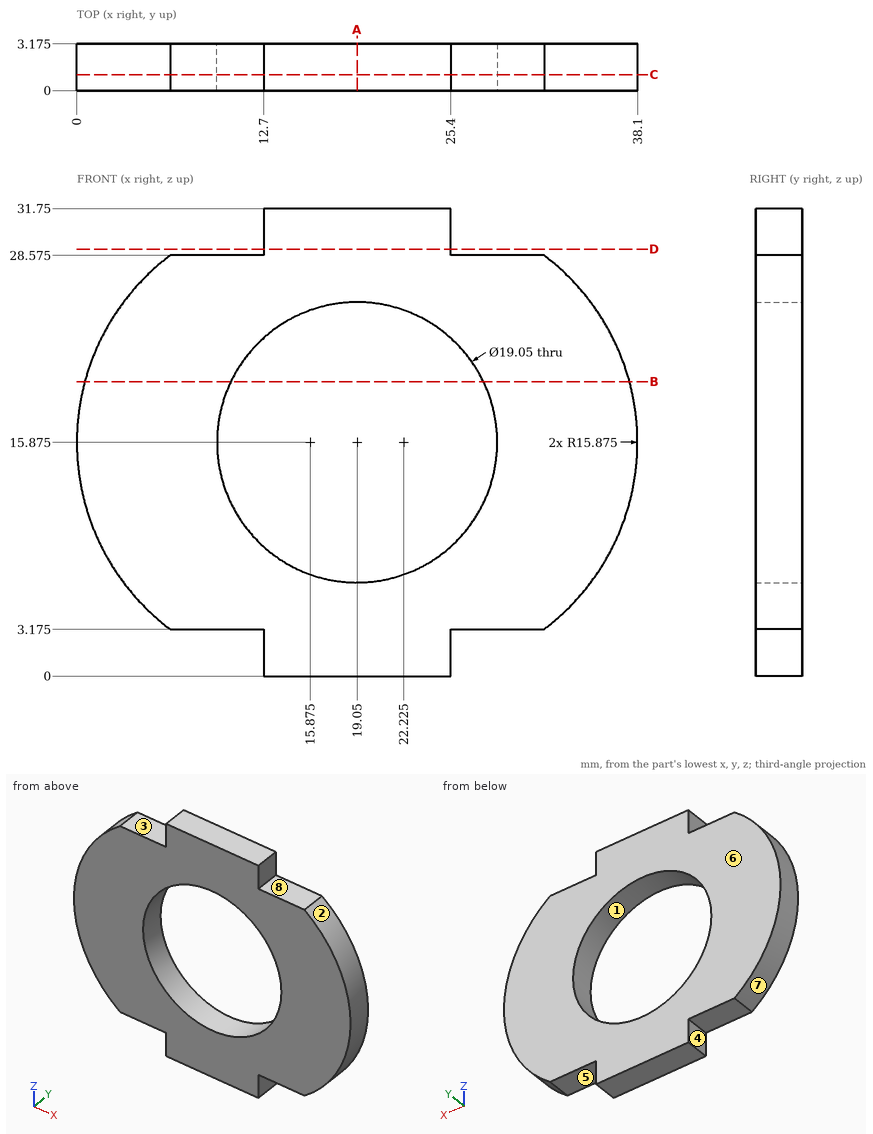
The drawing under review shows one solid part. Ordinate dimensions are in mm from its lowest x, y, z. A direction names the side the tool comes from. Coordinates: 2 decimals unless noted, no trailing zeros. Write each loop counter-clockwise with the first axis right and the second up, starting at its lowest first coordinate (ties: lowest second). Pieces come first, ordered by that corner, then holes. Notation, with made-up numbers: M 12.5,-19.5 L 30.5,-19.5 A35 ccw 30.5,13.5 Z; hole C -16,29 d1. An arc over 180 degrees is marked long. Put each result on its own line as item: value.
1) Clearance check with flat-ended pins moving along their axes: pin 1 Ø1 at (y, z) = (2, 18.5) entering from +X; pin 2 Ø1 at (x, y) = (10.5, 1.5) entering from +Z (3 decimals); pin 3 Ø1.5 at (x, z) = (33.5, 3.5) entering from -Y; pin 4 Ø1.6 at (x, y) = (8, 1.5) entering from -Z (3 decimals). State where each tip first meets the part, or that it passes through.
Computed:
pin 1: stops at x = 37.96
pin 2: stops at z = 28.575
pin 3: passes through
pin 4: stops at z = 3.175
2) Add section A-A on x = 19.05. Give the boundary of the cut face in (y, z) (3 decimals).
Computed:
outline: M 0,0 L 3.175,0 L 3.175,6.35 L 0,6.35 Z; M 0,25.4 L 3.175,25.4 L 3.175,31.75 L 0,31.75 Z
3) Wall thickness on probe 1 along Z at (x, y) = (19.05, 1.35); probe 2 along X at (y, z) = (2.2, 29.5); probe 3 along Z at (x, y) = (11.5, 0.4) (3 decimals): over which ranges is each line inside the solid? List them lowest first. Write a range as [from, to].
Computed:
probe 1: z = [0, 6.35], [25.4, 31.75]
probe 2: x = [12.7, 25.4]
probe 3: z = [3.175, 10.068], [21.682, 28.575]
4) Add section C-C on y = 1.1. Give the boundary of the cut face in (x, z) (3 decimals).
Computed:
outline: M 6.35,3.175 L 12.7,3.175 L 12.7,0 L 25.4,0 L 25.4,3.175 L 31.75,3.175 A15.875 ccw 31.75,28.575 L 25.4,28.575 L 25.4,31.75 L 12.7,31.75 L 12.7,28.575 L 6.35,28.575 A15.875 ccw Z; hole C 19.05,15.875 d19.05
5) Add section B-B on z = 20. Give the boundary of the cut face in (x, y) (3 decimals).
Computed:
outline: M 0.545,0 L 10.465,0 L 10.465,3.175 L 0.545,3.175 Z; M 27.635,0 L 37.555,0 L 37.555,3.175 L 27.635,3.175 Z
6) Add section D-D on z = 29. Give the boundary of the cut face in (x, y) (3 decimals).
Computed:
outline: M 12.7,0 L 25.4,0 L 25.4,3.175 L 12.7,3.175 Z
7) Draft analysis for pull direction Z (two halves, no side actions). For the marked faces 1, 2 and 3, state which applies: released by +Z, released by -Z, zero draft, split by the parting line, or undercut.
Computed:
face 1: undercut
face 2: split by the parting line
face 3: released by +Z
8) For the marked faces 4, 5, 6, 7 and 8, list the 3-axis set-ups (+Z, -Z, +X, -X, +Y, -Y) from which the entire face can be reached by the end or side of a thin tool; tool diameter is ignored.
Computed:
face 4: -Z, -X, +Y, -Y
face 5: -Z, +X, +Y, -Y
face 6: +Z, -Z, +X, -X, +Y
face 7: -X, +Y, -Y
face 8: +Z, +X, +Y, -Y
